Source: CAD feature listing. Evaluate the final solid. Frame: model axes, mm. A direction names the side the tool comes from. Give positions to 0.01 mm unless a question says otherwise; leave off trailing zeros. Loops run counter-clockwise (first coordinate to the right, second up) from the corner with the lowest first, then second, coordinate; pieces in that order, holes last. Notation, with made-up numbers: M 77,36.25 L 125,36.25 A17 ccw 125,64.25 Z; hole C 40,45 d10. An arc over 180 degrees is marked long. Answer in a Markdown table with one row per item.
```python
from build123d import *

# Parameters (mm, degrees)
SKETCH1_W                          = 55.88
SKETCH1_H                          = 55.88
BOSS_EXTRUDE1_DEPTH                = 9
F_1_4_0_25_CLEARANCE_DOWEL_HOLE1_D = 3.429
SKETCH4_W                          = 44.289451808
SKETCH4_H                          = 35.4
CUT_EXTRUDE1_DEPTH                 = 4
SKETCH5_W                          = 55.88
SKETCH5_H                          = 5
BOSS_EXTRUDE2_DEPTH                = 15.24
SKETCH6_W                          = 55.88
SKETCH6_H                          = 5
BOSS_EXTRUDE3_DEPTH                = 15.24
F_1_4_0_25_CLEARANCE_DOWEL_HOLE2_D = 6.499999954


with BuildPart() as part:
    # Sketch1 → Boss-Extrude1 (new body)
    with BuildSketch(Plane(origin=(0, 0, 0), x_dir=(1, 0, 0), z_dir=(0, 1, 0))):
        Rectangle(SKETCH1_W, SKETCH1_H)
    extrude(amount=BOSS_EXTRUDE1_DEPTH)

    # 1/4 (0.25) Clearance Dowel Hole1 (through all)
    with Locations(Plane(origin=(0, 9, 0), x_dir=(1, 0, 0), z_dir=(0, 1, 0))):
        with Locations((-17.144725904, -12.7), (-17.144725904, 12.7), (17.145, -12.837103678), (17.145, 12.562896322)):
            Hole(F_1_4_0_25_CLEARANCE_DOWEL_HOLE1_D / 2)

    # Sketch4 → Cut-Extrude1 (cut)
    with BuildSketch(Plane.XZ):
        Rectangle(SKETCH4_W, SKETCH4_H)
    extrude(amount=-CUT_EXTRUDE1_DEPTH, mode=Mode.SUBTRACT)

    # Sketch5 → Boss-Extrude2 (add)
    with BuildSketch(Plane.XY.offset(27.94)):
        with Locations((0, 2.5)):
            Rectangle(SKETCH5_W, SKETCH5_H)
    extrude(amount=BOSS_EXTRUDE2_DEPTH)

    # Sketch6 → Boss-Extrude3 (add)
    with BuildSketch(Plane(origin=(0, 0, -27.94), x_dir=(-1, 0, 0), z_dir=(0, 0, -1))):
        with Locations((0, 2.5)):
            Rectangle(SKETCH6_W, SKETCH6_H)
    extrude(amount=BOSS_EXTRUDE3_DEPTH)

    # 1/4 (0.25) Clearance Dowel Hole2 (through all)
    with Locations(Plane(origin=(0, 5, 0), x_dir=(1, 0, 0), z_dir=(0, 1, 0))):
        with Locations((11.43, 38.1), (-13.97, 38.1), (-13.97, -38.1), (11.43, -38.1)):
            Hole(F_1_4_0_25_CLEARANCE_DOWEL_HOLE2_D / 2)


solid = part.part
```
1) Section D-D, the plane x = -6.5. Return loops of the section in (y, z).
Reply:
| item | result |
|---|---|
| outline | M 0,-43.18 L 5,-43.18 L 5,-27.94 L 9,-27.94 L 9,27.94 L 5,27.94 L 5,43.18 L 0,43.18 L 0,17.7 L 4,17.7 L 4,-17.7 L 0,-17.7 Z |
2) Set-up query: faces 1 (the flat face through (0, 4, 0)), 2 (the cylindrical face through (-17.07, 2.47, 37.12)), 3 (the flat face through (0, 5, 35)). Return all of +Z, -Z, +X, -X, +Y, -Y with unobstructed straight access to the full face (end or side cutting, diameter ignored); none if empty.
Reply:
| item | result |
|---|---|
| face 1 | -Y |
| face 2 | +Y, -Y |
| face 3 | +Z, +X, -X, +Y |
3) Material intervals for L1, parallel to Z at x = 11.43, y = 2.1; L2, parallel to X at y = 2.8, z = -38.1; L3, parallel to X at y = 7.5, z = 13, sorted ascending.
Reply:
| item | result |
|---|---|
| L1 | z = -43.18 to -41.35, -34.85 to -17.7, 17.7 to 34.85, 41.35 to 43.18 |
| L2 | x = -27.94 to -17.22, -10.72 to 8.18, 14.68 to 27.94 |
| L3 | x = -27.94 to -18.83, -15.46 to 15.44, 18.85 to 27.94 |
4) Section C-C, the plane z = 38.1. Return loops of the section in (x, y), then the cut area to 3 significant figures.
Reply:
| item | result |
|---|---|
| outline | M -27.94,0 L -17.22,0 L -17.22,5 L -27.94,5 Z; M -10.72,0 L 8.18,0 L 8.18,5 L -10.72,5 Z; M 14.68,0 L 27.94,0 L 27.94,5 L 14.68,5 Z |
| area | 214 mm² |
5) Pin query (flat end, axial travel): pin 1 Ø8.5 at (x, z) = (11.43, 38.1) entering from +Y; pin 2 Ø5.5 at (x, z) = (17.14, -12.56) entering from -Y; pin 3 Ø2 at (x, y) = (0.5, 6.5) entering from -Z. Return the tip coordinate at first contact, or that it passes through.
Reply:
| item | result |
|---|---|
| pin 1 | stops at y = 5 |
| pin 2 | stops at y = 4 |
| pin 3 | stops at z = -27.94 |
6) Section B-B, the plane x = 11.43. Return loops of the section in (y, z), then the cut area to 3 significant figures.
Reply:
| item | result |
|---|---|
| outline | M 0,-43.18 L 5,-43.18 L 5,-41.35 L 0,-41.35 Z; M 0,-34.85 L 5,-34.85 L 5,-27.94 L 9,-27.94 L 9,27.94 L 5,27.94 L 5,34.85 L 0,34.85 L 0,17.7 L 4,17.7 L 4,-17.7 L 0,-17.7 Z; M 0,41.35 L 5,41.35 L 5,43.18 L 0,43.18 Z |
| area | 449 mm² |
7) Section A-A, the plane y = 2. Return loops of the section in (x, z).
Reply:
| item | result |
|---|---|
| outline | M -27.94,-43.18 L 27.94,-43.18 L 27.94,43.18 L -27.94,43.18 Z; hole M -22.14,-17.7 L 22.14,-17.7 L 22.14,17.7 L -22.14,17.7 Z; hole C -13.97,-38.1 d6.5; hole C -13.97,38.1 d6.5; hole C 11.43,-38.1 d6.5; hole C 11.43,38.1 d6.5 |
8) Pull-direction query (X, two-part tool) for faces 4 (the flat face through (0, 2, -17.7)), 5 (the flat face through (27.94, 3, 1)), 6 (the flat face through (0, 5, -35)), 7 (the flat face through (-27.94, 3, 1)); classes: released by +X, released by -X, zero draft, split by the parting line, or undercut.
Reply:
| item | result |
|---|---|
| face 4 | undercut |
| face 5 | released by +X |
| face 6 | zero draft |
| face 7 | released by -X |
